Autodesk Inventor part; units mm, degrees
ref_plane "YZ Plane" through (0, 0, 0) normal (1, 0, 0) x (0, 1, 0)
ref_plane "XZ Plane" through (0, 0, 0) normal (0, 1, 0) x (-1, 0, 0)
ref_plane "XY Plane" through (0, 0, 0) normal (0, 0, 1) x (1, 0, 0)
sketch "Sketch1" plane through (0, 0, 0) normal (0, 1, 0) x (-1, 0, 0)
  line L0 (-3, -30) -> (3, -30)
  line L1 (3, -30) -> (3, 30)
  line L2 (3, 30) -> (-3, 30)
  line L3 (-3, 30) -> (-3, -30)
  line L4 (-3, -30) -> (3, 30) construction
  line L5 (3, -30) -> (-3, 30) construction
  line L6 (3, 30) -> (3, 20)
  line L7 (3, 20) -> (28, 20)
  line L8 (28, 20) -> (28, 5)
  line L9 (28, 5) -> (3, 5)
  line L10 (3, 5) -> (3, 20)
  line L11 (15.5, 20) -> (10.5, 20)
  line L12 (15.5, 20) -> (8, 20)
  line L13 (3, 20) -> (8, 20)
  line L14 (8, 20) -> (8, 15)
  line L15 (8, 15) -> (3, 15)
  line L16 (3, 15) -> (3, 20)
  line L17 (3, 15) -> (23, 15)
  line L18 (23, 15) -> (23, 10)
  line L19 (23, 10) -> (3, 10)
  line L20 (3, 10) -> (3, 15)
  line L21 (0, 0) -> (20, 0)
  line L22 (3, -20) -> (28, -20)
  line L23 (28, -20) -> (28, -5)
  line L24 (28, -5) -> (3, -5)
  line L25 (8, -20) -> (8, -15)
  line L26 (8, -15) -> (3, -15)
  line L27 (3, -15) -> (23, -15)
  line L28 (23, -15) -> (23, -10)
  line L29 (23, -10) -> (3, -10)
  line L30 (8, 20) -> (3, 20)
  line L31 (3, 20) -> (3, 15)
  line L32 (3, 15) -> (8, 15)
  line L33 (8, 15) -> (8, 20)
  line L34 (8, -15) -> (3, -15)
  line L35 (3, -15) -> (3, -20)
  line L36 (3, -20) -> (8, -20)
  line L37 (8, -20) -> (8, -15)
  line L38 (28, 5) -> (28, -5)
  point P0 (8, 20)
  point P1 (8, 15)
  point P2 (3, 10)
  point P3 (3, -10)
  point P4 (8, -15)
  point P5 (3, -5)
  point P6 (3, 5)
  point P7 (28, -2.5)
  point P8 (23, -2.5)
  point P9 (23, -2.5)
  point P10 (23, 2.5)
  point P11 (23, 2.5)
  point P12 (28, 2.5)
  point P13 (3, 10)
  dimension "d0" = 6
  dimension "d1" = 60
  dimension "d2" = 10
  dimension "d3" = 25
  dimension "d4" = 15
  dimension "d8" = 5
  dimension "d9" = 5
  dimension "d10" = 20
  dimension "d11" = 5
  dimension "d12" = 20
extrude "Extrusion1" add sketch "Sketch1" along normal blind 15 contours L3 L2 L1 L0 | L25 L27 L28 L29 L1 L24 L23 L22 | L7 L8 L9 L1 L19 L18 L17 L14
sketch "Sketch2" plane through (-28, 0, 20) normal (0, 0, 1) x (1, 0, 0)
  line L0 (20, 0) -> (20, 15)
  line L1 (20, 7.5) -> (12.5, 7.5)
  circle A0 centre (12.5, 7.5) radius 3
  point P0 (28, 0)
  dimension "d15" = 7.5
  dimension "d16" = 6
extrude "Extrusion2" cut sketch "Sketch2" against normal through all
fillet "Fillet1" radius 2 16 edges at (-8, 7.5, 20) (-8, 7.5, 15) (-3, 7.5, 10) (-28, 7.5, 20) (-28, 7.5, 5) (-23, 7.5, 10) (-23, 7.5, 15) (-23, 7.5, -15) (-23, 7.5, -10) (-28, 7.5, -5) (-28, 7.5, -20) (-8, 7.5, -20) (-8, 7.5, -15) (-3, 7.5, -10) (-3, 7.5, 5) (-3, 7.5, -5)
sketch "Sketch3" plane through (-3, 0, -30) normal (-1, 0, 0) x (0, 0, 1)
  line L0 (60, 0) -> (60, 15)
  line L1 (60, 7.5) -> (55, 7.5)
  line L2 (0, 0) -> (0, 15)
  line L3 (0, 7.5) -> (5, 7.5)
  circle A0 centre (55, 7.5) radius 3
  circle A1 centre (5, 7.5) radius 3
  point P0 (30, 0)
  dimension "d20" = 5
  dimension "d21" = 5
  dimension "d22" = 6
  dimension "d23" = 6
extrude "Extrusion3" cut sketch "Sketch3" against normal through all
fillet "Fillet2" radius 3 4 edges at (0, 15, 30) (0, 15, -30) (0, 0, -30) (0, 0, 30)
properties part number "Festoon_Carriage"
Can you work these out from the model? Positions are in its coordinate system, mm. A direction names the side the tool comes from. Coordinates: 2 decimals unless noted, no trailing zeros. Order: outer loops, then holes, each group sorted by start corner. A loop starts at its lowest first (then second) coordinate and runs counter-clockwise, first axis right, second up. Notation, with made-up numbers: M 16.5,44.5 L 71.5,44.5 A22 ccw 71.5,61.5 Z; hole C -16,0.5 d1. An arc over 180 degrees is marked long. Write item = value, one per line.
(1) Suppose I cut it at D-D on z = 25. Please give me the cut outline in (x, y), plus the area to 3 significant figures.
Results are:
outline = M -3,0 L 3,0 L 3,4.5 L -3,4.5 Z; M -3,10.5 L 3,10.5 L 3,15 L -3,15 Z
area = 54.0 mm2
(2) For faces 1 (the face through (-8.57, 7.6, -19.4)), 2 (the face through (-8.6, 7.6, -15.57)), 3 (the face through (-20, 7, 20)), which set-ups out of +Z, -Z, +X, -X, +Y, -Y let a thin tool reach every point of the face, with its end or its side?
Results are:
face_1 = -Z, +Y, -Y
face_2 = +Y, -Y
face_3 = +Z, -X, +Y, -Y
(3) I need wall thicknesses on line 1 along Z through (x, y) = (-17.5, 1); line 2 along X through (y, z) = (7, -12); line 3 along Z through (x, y) = (-24.5, 13). Which ranges of each line are inside material? Lowest first, please. Write a range as [from, to].
Results are:
line_1 = [-20, -15], [-10, -5], [5, 10], [15, 20]
line_2 = [-28, -23], [-3, 3]
line_3 = [-20, -5], [5, 20]
(4) For pin 1 Ø5.5 at (x, y) = (-15.5, 7.5) entering from +Z; pin 2 Ø5 at (x, y) = (-17.5, 12.5) entering from -Z; pin 3 Ø2 at (y, z) = (11, -6.5) entering from -X; pin 4 Ø7.5 at (x, y) = (-16.5, 8) entering from +Z, each with a flat end and sliding along its axis, tell me the tip position at first contact or that it passes through.
Results are:
pin_1 = through
pin_2 = -20
pin_3 = -28
pin_4 = 20
(5) Suppose I cut it at B-B on x = -20. Please give me the cut outline in (y, z).
Results are:
outline = M 0,-20 L 15,-20 L 15,-15 L 0,-15 Z; M 0,-10 L 15,-10 L 15,-5 L 0,-5 Z; M 0,5 L 15,5 L 15,10 L 0,10 Z; M 0,15 L 15,15 L 15,20 L 0,20 Z
(6) Suppose I cut it at C-C on z = -9. Please give me the cut outline in (x, y).
Results are:
outline = M -28,0 L 3,0 L 3,15 L -28,15 Z; hole C -15.5,7.5 d6
(7) If we mould it in two halves opening along Y, with no side actions, what happens to faces 4 (the face through (-18.5, 7.6, 7.5)), 5 (the face through (-15, 4, 15)), 6 (the face through (-0.04, 0.9, -29.14)), 7 (the face through (-12, 15, -6))? For each: pulls with the +Y half, pulls with the -Y half, needs draft (parallel to the pull), parting line crosses it, or undercut.
Results are:
face_4 = undercut
face_5 = needs draft
face_6 = pulls with the -Y half
face_7 = pulls with the +Y half
(8) Suppose I cut it at A-A on x = -15.5. State how many separate pieces and enclosed holes the cut face has, plus the area to 3 significant figures.
Results are:
separate_pieces = 8
enclosed_holes = 0
area = 180 mm2
